```python
from build123d import *

# Parameters (mm, degrees)
SKETCH1_R           = 75
BOSS_EXTRUDE1_DEPTH = 7
SKETCH2_R           = 2.5
BOSS_EXTRUDE2_DEPTH = 20
CIRPATTERN1_COUNT   = 4
CIRPATTERN3_COUNT   = 4


# Read off the part's stored shape, not the designer's step: Dome1
with BuildPart() as part:
    # Sketch1 → Boss-Extrude1 (new body)
    with BuildSketch(Plane(origin=(0, 0, 0), x_dir=(1, 0, 0), z_dir=(0, 1, 0))):
        with Locations(Location((0, 0, 0), (0, 0, 270))):
            Circle(SKETCH1_R)
    extrude(amount=BOSS_EXTRUDE1_DEPTH)

    # Sketch2 → Boss-Extrude2 (add)
    with BuildSketch(Plane(origin=(0, 7, 0), x_dir=(1, 0, 0), z_dir=(0, 1, 0))):
        with Locations(Location((35, 35, 0), (0, 0, 270))):
            Circle(SKETCH2_R)
    boss_extrude2 = extrude(amount=BOSS_EXTRUDE2_DEPTH)

    # CirPattern1: Boss-Extrude2 ×4 about axis
    cirpattern1_axis = Axis((0, 0, 0), (0, 1, 0))
    for i in range(1, CIRPATTERN1_COUNT):
        add(boss_extrude2.rotate(cirpattern1_axis, i * 360 / CIRPATTERN1_COUNT))

    # Dome1 outline → Dome1 (revolve)
    with BuildSketch(Plane(origin=(-35, 0, -35), x_dir=(1, 0, 0), z_dir=(0, 0, 1))):
        with BuildLine():
            Line((0, 27), (2.5, 26.999999997))
            ThreePointArc((2.5, 26.999999997), (1.767766954, 28.767766952), (0, 29.5))
            Line((0, 29.5), (0, 27))
        make_face()
    dome1 = revolve(axis=Axis((-35, 0, -35), (0, 1, 0)))

    # CirPattern3: Dome1 ×4 about axis
    cirpattern3_axis = Axis((0, 0, 0), (0, 1, 0))
    for i in range(1, CIRPATTERN3_COUNT):
        add(dome1.rotate(cirpattern3_axis, i * 360 / CIRPATTERN3_COUNT))


solid = part.part
```
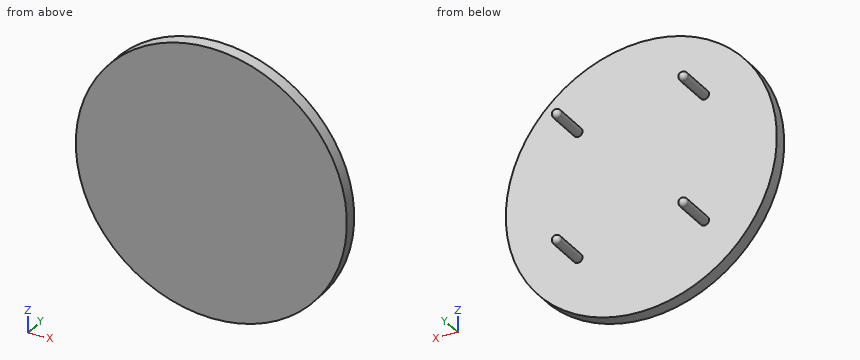
Design review of the part built by this model. Coordinates are the model's own, in mm. Give positions to 0.01 mm unless a question says otherwise; leave off trailing zeros. Order: outer loops, then holes, each group sorted by start corner. A loop starts at its lowest first (then second) coordinate and runs counter-clockwise, first axis right, second up. Notation, with made-up numbers: (73, 60.25) - (113, 60.25) arc R24 cw to (113, 99.25) - close; hole circle Ø6 at (4.5, 37). An arc over 180 degrees is marked (long way). Use a Markdown table: item, result. Add a question column.
(1) Add section D-D on z = 60. Give the boundary of the cut face in (x, y).
(2) Add section A-A on z = -35. Give the boundary of the cut face in (x, y).
(3) Clearance check with flat-ended pins moving along their axes: P1, Ø4, axis at x = 48.5, z = -49, coming from the +Y side; P2, Ø1.5, axis at y = 22, z = 35, coming from the -X side; P3, Ø3, axis at y = 5.5, z = 50.5, coming from the +X side. State where each tip first meets the part, or that it passes through.
(4) Add section B-B on y = 9. Give the boundary of the cut face in (x, z).
(5) Wall thickness on probe 1 along Y at (x, z) = (7, -65.5); probe 2 along Z at (x, y) = (33.5, 26.5); probe 3 along Z at (x, y) = (-33, 22.5): over which ranges is each line inside the solid? List them lowest first. Write a range as [from, to].
(6) Add section C-C on x = 0. Give the boundary of the cut face in (y, z), then the cut area to 3 significant figures.
Report:
| question | item | result |
|---|---|---|
| 1 | outline | (-45, 0) - (45, 0) - (45, 7) - (-45, 7) - close |
| 2 | outline | (-66.33, 0) - (66.33, 0) - (66.33, 7) - (37.5, 7) - (37.5, 27) arc R2.5 ccw to (32.5, 27) - (32.5, 7) - (-32.5, 7) - (-32.5, 27) arc R2.5 ccw to (-37.5, 27) - (-37.5, 7) - (-66.33, 7) - close |
| 3 | P1 | stops at y = 7 |
| 3 | P2 | stops at x = -37.5 |
| 3 | P3 | stops at x = 56.78 |
| 4 | outline | circle Ø5 at (-35, -35); circle Ø5 at (-35, 35); circle Ø5 at (35, -35); circle Ø5 at (35, 35) |
| 5 | probe 1 | y = [0, 7] |
| 5 | probe 2 | z = [-37, -33], [33, 37] |
| 5 | probe 3 | z = [-36.5, -33.5], [33.5, 36.5] |
| 6 | outline | (0, -75) - (7, -75) - (7, 75) - (0, 75) - close |
| 6 | area | 1,050 mm² |
